Source: CAD feature listing. Evaluate the final solid. Frame: model axes, mm. Give positions to 0.01 mm unless a question says otherwise; leave off trailing zeros. Order: outer loops, then holes, each group sorted by start corner. A loop starts at its lowest first (then second) coordinate and runs counter-clockwise, first axis right, second up. Notation, with made-up numbers: (74.25, 32.5) - (129.25, 32.5) arc R12 ccw to (129.25, 45.5) - close; hole circle Ø8 at (53.5, -35.5). An arc over 180 degrees is marked (long way). Answer as CSV lines item,"result".
```python
from build123d import *

# Parameters (mm, degrees)
SKIZZE1_W                       = 19.2
SKIZZE1_H                       = 70
SKIZZE1_W_2                     = 263
SKIZZE1_H_2                     = 146.4
SKIZZE1_W_3                     = 14.2
AUFSATZ_LINEAR_AUSTRAGEN1_DEPTH = 5


with BuildPart() as part:
    # Skizze1 → Aufsatz-Linear austragen1 (new body)
    with BuildSketch(Plane(origin=(0, 15, 0), x_dir=(1, 0, 0), z_dir=(0, 1, 0))):
        with Locations((-138.6, 0)):
            Rectangle(SKIZZE1_W, SKIZZE1_H)
        with Locations((2.5, 0)):
            Rectangle(SKIZZE1_W_2, SKIZZE1_H_2)
        with Locations((141.1, 0)):
            Rectangle(SKIZZE1_W_3, SKIZZE1_H)
    extrude(amount=AUFSATZ_LINEAR_AUSTRAGEN1_DEPTH)


solid = part.part
```
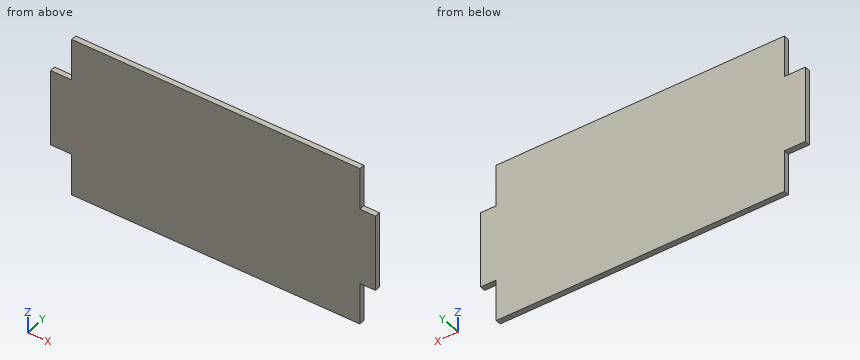
(1) Cut plane A-A (y = 18.45). Return loops of the section in (x, z).
Completed:
outline,"(-148.2, -35) - (-129, -35) - (-129, -73.2) - (134, -73.2) - (134, -35) - (148.2, -35) - (148.2, 35) - (134, 35) - (134, 73.2) - (-129, 73.2) - (-129, 35) - (-148.2, 35) - close"
(2) Cut plane B-B (z = -48). Return loops of the section in (x, y).
Completed:
outline,"(-129, 15) - (134, 15) - (134, 20) - (-129, 20) - close"
(3) Ray query, line 1 (Z direction, x = -135.5, y = 19.7); line 2 (X direction, y = 16.15, z = -64). Return the intervals inside material, ascending. Write a range as from..to.
Completed:
line 1,"-35..35"
line 2,"-129..134"
(4) Contact query for flat-ended pins moving along their axis: pin 1 (2.5 mm diameter, centred on x = -136, y = 18, fed in from -Z); pin 2 (2.5 mm diameter, centred on y = 18, z = 52, fed in from +X); pin 3 (2.5 mm diameter, centred on x = 140.5, y = 17.5, fed in from +Z). Output: stop coordinate, or through.
Completed:
pin 1,"z = -35"
pin 2,"x = 134"
pin 3,"z = 35"
